Work out the finished part from the listing and answer in its coordinate system (mm). Face numbers are marked on the shaded views. Round coordinates to 2 decimals unless told otherwise and drop trailing zeros. Write each loop counter-clockwise with the first axis right and the second up, starting at its lowest first coordinate (ties: lowest second). Pieces come first, ordered by that corner, then holes.
1. Flat-ended cylindrical pins translate along their axes: pin 1 Ø1 at (y, z) = (-0.5, 1.5) entering from -X; pin 2 Ø1.2 at (x, z) = (0, 0) entering from +Y; pin 3 Ø1.5 at (x, y) = (-0.5, 0.5) entering from +Z. Find the tip coordinate at first contact, or state that the pin passes through.
2. Find section B-B (z = 0.5). Write down the section's boundary in (x, y).
3. Determine the mould class of the marked faces 1, 2 and 3 for opening direction Z: pulls with the +Z half, pulls with the -Z half, needs draft (parallel to the pull), parting line crosses it, or undercut.
4. Find section C-C (y = 0). Write down the section's boundary in (x, z).
5. Straight lines are drawn through the part: probe 1 along X at (y, z) = (0.8, 0); probe 2 along Z at (x, y) = (0, 0.8); probe 3 along X at (y, z) = (0.35, -0.5). For each, find the intervals that lie inside material, in ascending order.
6. Find section A-A (x = 0). Write down the section's boundary in (y, z), and give its area (3 significant figures).
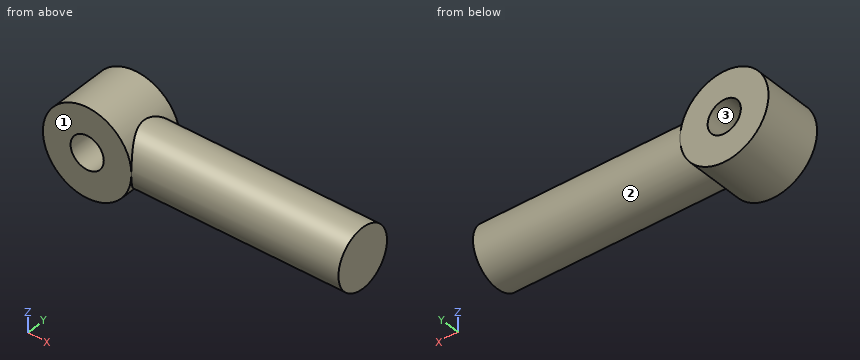
```python
from build123d import *

# Parameters (mm, degrees)
SKETCH1_R                = 1.35
BOSS_EXTRUDE1_DEPTH      = 11.35
BOSS_EXTRUDE2_DEPTH      = 1.35
BOSS_EXTRUDE2_DEPTH_BACK = 1.35
SKETCH2_R                = 2
SKETCH3_R                = 0.75
CUT_EXTRUDE1_DEPTH       = 11.35


with BuildPart() as part:
    # Sketch1 → Boss-Extrude1 (new body)
    with BuildSketch(Plane(origin=(0, 0, 0), x_dir=(0, 0, -1), z_dir=(1, 0, 0))):
        Circle(SKETCH1_R)
    extrude(amount=BOSS_EXTRUDE1_DEPTH)

    # Sketch2 → Boss-Extrude2 (add, two sides: drawn at the far end of the back side and taken through both)
    with BuildSketch(Plane(origin=(0, 0, 0), x_dir=(1, 0, 0), z_dir=(0, 1, 0)).offset(-BOSS_EXTRUDE2_DEPTH_BACK)):
        Circle(SKETCH2_R)
    extrude(amount=BOSS_EXTRUDE2_DEPTH + BOSS_EXTRUDE2_DEPTH_BACK)

    # Sketch3 → Cut-Extrude1 (cut)
    with BuildSketch(Plane(origin=(0, 1.35, 0), x_dir=(1, 0, 0), z_dir=(0, 1, 0))):
        with Locations(Location((0, 0, 0), (0, 0, 270))):
            Circle(SKETCH3_R)
    extrude(amount=-CUT_EXTRUDE1_DEPTH, mode=Mode.SUBTRACT)


solid = part.part
```
Worked answers:
1. pin 1: stops at x = -1.73
1. pin 2: passes through
1. pin 3: stops at z = 2
2. outline: (-1.94, -1.35) - (-0.56, -1.35) - (-0.56, 1.35) - (-1.94, 1.35) - close; (0.56, -1.35) - (1.94, -1.35) - (1.94, -1.25) - (11.35, -1.25) - (11.35, 1.25) - (1.94, 1.25) - (1.94, 1.35) - (0.56, 1.35) - close
3. face 1: needs draft
3. face 2: parting line crosses it
3. face 3: undercut
4. outline: (1.48, -1.35) - (11.35, -1.35) - (11.35, 1.35) - (1.48, 1.35) arc R2 ccw (long way) to start; hole circle Ø1.5 at (0, 0)
5. probe 1: x = -2 to -0.75, 0.75 to 11.35
5. probe 2: z = -2 to -0.75, 0.75 to 2
5. probe 3: x = -1.94 to -0.56, 0.56 to 11.35
6. outline: (-1.35, -2) - (1.35, -2) - (1.35, -0.75) - (-1.35, -0.75) - close; (-1.35, 0.75) - (1.35, 0.75) - (1.35, 2) - (-1.35, 2) - close
6. area: 6.75 mm2
